The model under review builds one solid part; all positions refer to its coordinate system, in mm. A direction names the side the tool comes from. Coordinates: 2 decimals unless noted, no trailing zeros. One line per question, with ' | ' between items. Start each with the question number.
from build123d import *

# Parameters (mm, degrees)
SKETCH1_W           = 140
SKETCH1_H           = 200
BOSS_EXTRUDE1_DEPTH = 4
SKETCH2_W           = 78
SKETCH2_H           = 2.05
SKETCH2_R           = 1.5
SKETCH2_H_2         = 5
CUT_EXTRUDE3_DEPTH  = 123.131077126
SKETCH3_W           = 6
SKETCH3_H           = 4
SKETCH3_R           = 1.5
CUT_EXTRUDE5_DEPTH  = 123.131077126
SKETCH4_R           = 1.5
CUT_EXTRUDE6_DEPTH  = 123.131077126
SKETCH6_W           = 3.05
SKETCH6_H           = 35
SKETCH6_W_2         = 4
SKETCH6_H_2         = 22
CUT_EXTRUDE13_DEPTH = 4
SKETCH7_R           = 1.5
CUT_EXTRUDE15_DEPTH = 123.131077126
SKETCH8_R           = 1.5
SKETCH8_W           = 2
SKETCH8_H           = 50
SKETCH8_W_2         = 25
SKETCH8_H_2         = 2.05
CUT_EXTRUDE16_DEPTH = 4


with BuildPart() as part:
    # Sketch1 → Boss-Extrude1 (new body)
    with BuildSketch(Plane(origin=(0, 0, 0), x_dir=(1, 0, 0), z_dir=(0, 1, 0))):
        Rectangle(SKETCH1_W, SKETCH1_H)
    extrude(amount=BOSS_EXTRUDE1_DEPTH)

    # Sketch2 → Cut-Extrude3 (cut, through all)
    with BuildSketch(Plane(origin=(0, 4, 0), x_dir=(1, 0, 0), z_dir=(0, 1, 0))):
        with Locations((0, 93.975)):
            Rectangle(SKETCH2_W, SKETCH2_H)
        with Locations(Location((-37.150844364, 90, 0), (0, 0, 270))):
            Circle(SKETCH2_R)
        with Locations(Location((37.150844364, 90, 0), (0, 0, 270))):
            Circle(SKETCH2_R)
        with Locations((0, 84.5)):
            Rectangle(SKETCH2_W, SKETCH2_H_2)
    extrude(amount=-CUT_EXTRUDE3_DEPTH, mode=Mode.SUBTRACT)

    # Sketch3 → Cut-Extrude5 (cut, through all)
    with BuildSketch(Plane(origin=(0, 4, 0), x_dir=(1, 0, 0), z_dir=(0, 1, 0))):
        with Locations((-64, 53)):
            Rectangle(SKETCH3_W, SKETCH3_H)
        with Locations(Location((65.055984274, 70, 0), (0, 0, 270))):
            Circle(SKETCH3_R)
        with Locations((64, 53)):
            Rectangle(SKETCH3_W, SKETCH3_H)
        with Locations(Location((-65.055984274, 70, 0), (0, 0, 270))):
            Circle(SKETCH3_R)
    extrude(amount=-CUT_EXTRUDE5_DEPTH, mode=Mode.SUBTRACT)

    # Sketch4 → Cut-Extrude6 (cut, through all)
    with BuildSketch(Plane(origin=(0, 4, 0), x_dir=(1, 0, 0), z_dir=(0, 1, 0))):
        with Locations(Location((59.5, 92, 0), (0, 0, 270))):
            Circle(SKETCH4_R)
        with Locations(Location((-59.5, 92, 0), (0, 0, 270))):
            Circle(SKETCH4_R)
        with Locations(Location((-46, 92, 0), (0, 0, 270))):
            Circle(SKETCH4_R)
        with Locations(Location((46, 92, 0), (0, 0, 90))):
            Circle(SKETCH4_R)
    extrude(amount=-CUT_EXTRUDE6_DEPTH, mode=Mode.SUBTRACT)

    # Sketch6 → Cut-Extrude13 (cut)
    with BuildSketch(Plane(origin=(0, 4, 0), x_dir=(1, 0, 0), z_dir=(0, 1, 0))):
        with Locations((13.525, 58.5)):
            Rectangle(SKETCH6_W, SKETCH6_H)
        with Locations((-8, 60)):
            Rectangle(SKETCH6_W_2, SKETCH6_H_2)
    extrude(amount=-CUT_EXTRUDE13_DEPTH, mode=Mode.SUBTRACT)

    # Sketch7 → Cut-Extrude15 (cut, through all)
    with BuildSketch(Plane(origin=(0, 4, 0), x_dir=(1, 0, 0), z_dir=(0, 1, 0))):
        with Locations(Location((27.764169226, -20.235830774, 0), (0, 0, 270))):
            Circle(SKETCH7_R)
        with Locations(Location((-27.764169226, -75.764169226, 0), (0, 0, 270))):
            Circle(SKETCH7_R)
        with Locations(Location((27.764169226, -75.764169226, 0), (0, 0, 270))):
            Circle(SKETCH7_R)
        with Locations(Location((24, 32.5, 0), (0, 0, 270))):
            Circle(SKETCH7_R)
        with Locations(Location((3, 1.5, 0), (0, 0, 270))):
            Circle(SKETCH7_R)
        with Locations(Location((-24, 1.5, 0), (0, 0, 270))):
            Circle(SKETCH7_R)
        with Locations(Location((-3, 32.5, 0), (0, 0, 270))):
            Circle(SKETCH7_R)
        with Locations(Location((-27.764169226, -20.235830774, 0), (0, 0, 270))):
            Circle(SKETCH7_R)
    extrude(amount=-CUT_EXTRUDE15_DEPTH, mode=Mode.SUBTRACT)

    # Sketch8 → Cut-Extrude16 (cut)
    with BuildSketch(Plane(origin=(0, 4, 0), x_dir=(1, 0, 0), z_dir=(0, 1, 0))):
        with Locations(Location((0, -10, 0), (0, 0, 270))):
            Circle(SKETCH8_R)
        with Locations(Location((-60, -90, 0), (0, 0, 270))):
            Circle(SKETCH8_R)
        with Locations(Location((60, -90, 0), (0, 0, 90))):
            Circle(SKETCH8_R)
        with Locations((-64.456694017, 0)):
            Rectangle(SKETCH8_W, SKETCH8_H)
        with Locations((64.456694017, 0)):
            Rectangle(SKETCH8_W, SKETCH8_H)
        with Locations((27.5, -93.975)):
            Rectangle(SKETCH8_W_2, SKETCH8_H_2)
        with Locations((-27.5, -93.975)):
            Rectangle(SKETCH8_W_2, SKETCH8_H_2)
    extrude(amount=-CUT_EXTRUDE16_DEPTH, mode=Mode.SUBTRACT)


solid = part.part
1) Wall thickness on L1, parallel to X at y = 1, z = -32.5; L2, parallel to Z at x = 8, y = 3.4; L3, parallel to X at y = 2.3, z = -63.5: over which ranges is each line inside the solid? List them lowest first.
2) Mouldability with a two-part tool opening along X and no side actions: class faces 1 (the face through (-1, 4, -1)), 2 (the face through (-64, 2, -51)) as +X half, -X half, draft (parallel to the pull), parting line (faces both ways), or undercut.
3) Machinability: for faces 3 (the face through (-1, 2, 100)), 4 (the face through (39, 2, -84)), which of the approach directions +Z, -Z, +X, -X, +Y, -Y give a long, thin tool a straight path to every point of the face, cutting with its end or side? Answer none if there is none.
4) Consider section A-A, the plane y = 1.6. Give the number of separate pieces and of enclosed holes in the cut face, plus the area to 3 significant figures.
5) Insertion check: pin 1 Ø2.5 at (x, z) = (-24, -1.5) entering from -Y. The pin has a flat end and moves straight along its axis. Give the tip position at first contact, or say it passes through.
Filled sheet:
1) L1: -70 to -4.5, -1.5 to 22.5, 25.5 to 70 | L2: -100 to -95, -92.95 to -87, -82 to 100 | L3: -70 to -10, -6 to 12, 15.05 to 70
2) face 1: draft | face 2: undercut
3) face 3: +Z, +X, -X, +Y, -Y | face 4: +Y, -Y
4) separate pieces: 1 | enclosed holes: 29 | area: 26,800 mm^2
5) pin 1: through
